```python
from build123d import *

# Parameters (mm, degrees)
F5_DEPTH  = 5
F3_R      = 20
F2_R      = 25
F2_R_2    = 20
F6_DEPTH  = 50
F7_DEPTH  = 10
F0_R      = 5
F0_R_2    = 2.5
F8_DEPTH  = 5
F9_DEPTH  = 25
F10_R     = 17.5
F11_DEPTH = 40
F12_DEPTH = 5
F13_R     = 5
F14_R     = 5


with BuildPart() as f5:
    # F1 (on Top) → F5 (new body)
    with BuildSketch(Plane.XY):
        with BuildLine():
            ThreePointArc((55.0272203653, -51.5364989145), (41.1164714576, 9.8481618987), (0, 57.5033955377))
            ThreePointArc((0, 57.5033955377), (-41.1164714576, 9.8481618987), (-55.0272203653, -51.5364989145))
            ThreePointArc((-55.0272203653, -51.5364989145), (0, -63.7570226936), (55.0272203653, -51.5364989145))
        make_face()
        with BuildLine():
            ThreePointArc((-45, -45), (-32.3889723065, 4.9444861533), (0, 45))
            ThreePointArc((0, 45), (32.3889723065, 4.9444861533), (45, -45))
            ThreePointArc((45, -45), (0, -53.7570226936), (-45, -45))
        make_face(mode=Mode.SUBTRACT)
        with BuildLine():
            ThreePointArc((45, -45), (32.3889723065, 4.9444861533), (0, 45))
            ThreePointArc((0, 45), (-32.3889723065, 4.9444861533), (-45, -45))
            ThreePointArc((-45, -45), (0, -53.7570226936), (45, -45))
        make_face()
    extrude(amount=F5_DEPTH)

    # F3 (on Top) + F2 (on Top) → F6 (join)
    with BuildSketch(Plane.XY):
        with Locations((0, 6.2429773064)):
            Circle(F3_R)
    with BuildSketch(Plane.XY):
        with Locations((0, -23.7570226936)):
            Circle(F2_R)
        with Locations((0, -23.7570226936)):
            Circle(F2_R_2, mode=Mode.SUBTRACT)
        with Locations((0, -23.7570226936)):
            Circle(F2_R_2)
    extrude(amount=F6_DEPTH)

    # F4 (on Top) → F7 (join)
    with BuildSketch(Plane.XY):
        Polygon((52.5, -37.5), (0, -37.5), (-52.5, -37.5), (-52.5, -52.5), (52.5, -52.5), align=None)
        Polygon((-7.5, 10.6258387864), (0, 10.6258387864), (7.5, 10.6258387864), (7.5, 50.6258387864), (-7.5, 50.6258387864), align=None)
    extrude(amount=F7_DEPTH)

    # F0 (on Top) → F8 (cut)
    with BuildSketch(Plane.XY):
        with Locations((-45, -45)):
            Circle(F0_R)
        with Locations((-45, -45)):
            Circle(F0_R_2, mode=Mode.SUBTRACT)
        with Locations((0, 45)):
            Circle(F0_R)
        with Locations((0, 45)):
            Circle(F0_R_2, mode=Mode.SUBTRACT)
        with Locations((45, -45)):
            Circle(F0_R)
        with Locations((45, -45)):
            Circle(F0_R_2, mode=Mode.SUBTRACT)
    extrude(amount=F8_DEPTH, mode=Mode.SUBTRACT)

    # F0 (on Top) → F9 (cut)
    with BuildSketch(Plane.XY):
        with Locations((-45, -45)):
            Circle(F0_R_2)
        with Locations((0, 45)):
            Circle(F0_R_2)
        with Locations((45, -45)):
            Circle(F0_R_2)
    extrude(amount=F9_DEPTH, mode=Mode.SUBTRACT)

    # F10 (on face) + F2 (on Top) → F11 (cut)
    with BuildSketch(Plane.XY):
        with Locations((0, 6.2429773064)):
            Circle(F10_R)
    with BuildSketch(Plane.XY):
        with Locations((0, -23.7570226936)):
            Circle(F2_R_2)
    extrude(amount=F11_DEPTH, mode=Mode.SUBTRACT)

    # F12 (cut): a face of the model
    f12_faces = [f5.faces().sort_by_distance(p)[0] for p in [
        (0, -12.7665147671, 50),
    ]]
    extrude(f12_faces, amount=-F12_DEPTH, mode=Mode.SUBTRACT)

    # F13
    f13_edges = [f5.edges().sort_by_distance(p)[0] for p in [
        (52.5, -52.5, 7.5),
        (52.5, -37.5, 7.5),
        (55.02722, -51.536499, 2.5),
        (-55.02722, -51.536499, 2.5),
        (-52.5, -52.5, 7.5),
        (-52.5, -37.5, 7.5),
        (-7.5, 50.625839, 7.5),
        (0, 57.503396, 2.5),
        (7.5, 50.625839, 7.5),
    ]]
    fillet(f13_edges, radius=F13_R)

    # F14
    f14_edges = [f5.edges().sort_by_distance(p)[0] for p in [
        (19.138968, 12.04814, 5),
        (-24.779157, -20.441394, 5),
        (24.779157, -20.441394, 5),
        (-19.138968, 12.04814, 5),
        (-16.535946, -5.007023, 25),
        (16.535946, -5.007023, 25),
        (0, 26.242977, 45),
        (0, -48.757023, 45),
    ]]
    fillet(f14_edges, radius=F14_R)


solid = f5.part
```
CAD build for the part. Positions are in the model's coordinates, mm. A direction names the side the tool comes from. Round coordinates to 2 decimals unless told otherwise and drop trailing zeros. Write each loop counter-clockwise with the first axis right and the second up, starting at its lowest first coordinate (ties: lowest second). Pieces come first, ordered by that corner, then holes. Notation, with made-up numbers: M 68,-3 L 78,-3 A21 cw 78,15 Z; hole C 49.5,15.25 d1. An arc over 180 degrees is marked long. One line per question, with ' | ' between items.
1. Probe L1, parallel to X at y = -45, z = 8; L2, parallel to Y at x = 0, z = 1; L3, parallel to Y at x = 0, z = 8.95. List the from-to ranges inside material, lowest first. Write a range as from..to.
Working result:
L1: -52.5..-47.5, -42.5..42.5, 47.5..52.5 | L2: -63.76..-43.76, 23.74..40, 50..56.32 | L3: -52.5..-43.76, 23.74..42.5, 47.5..50.63
2. Which spindle directions (+Z, -Z, +X, -X, +Y, -Y) get a long thin tool onto all of the face, cutting with end or side? Do faces 4 (the cylindrical face through (41, -42, 2)), 5 (the cylindrical face through (51, -51.07, 7.54)), 6 (the cylindrical face through (-0.799, -48.744, 24.79)), 7 (the cylindrical face through (-5.996, 49.2, 7.535)), 8 (the cylindrical face through (-51.07, -51, 7.54)). Say none if no direction does.
Working result:
face 4: -Z | face 5: +Z, +X, -Y | face 6: +Z | face 7: +Z, -X, +Y | face 8: +Z, -X, -Y
3. Cut at B-B on x = -32.5. Write the cut outline in (y, z), and give its area (3 significant figures).
Working result:
outline: M -59.63,0 L 24.46,0 L 24.46,5 L -37.5,5 L -37.5,10 L -52.5,10 L -52.5,5 L -59.63,5 Z | area: 495 mm2
4. Mould opens along Y. For faces 1 (the flat face through (-7.5, 35, 7)), 2 (the cylindrical face through (-51, -38.93, 7.54)), 3 (the flat face through (34, -37.5, 7)) say: pulls with the +Y half, pulls with the -Y half, needs draft (parallel to the pull), parting line crosses it, or undercut.
Working result:
face 1: needs draft | face 2: pulls with the +Y half | face 3: undercut
5. Pin check, flat tips, straight feed: pin 1 Ø12 at (x, y) = (2, -19) entering from -Z; pin 2 Ø6 at (x, y) = (-45, -45) entering from -Z; pin 3 Ø2 at (x, z) = (-13.5, 28.5) entering from +Y; pin 4 Ø3 at (x, y) = (-45, -45) entering from -Z. Stop position of each tip, or through.
Working result:
pin 1: z = 40 | pin 2: z = 5 | pin 3: y = 21.86 | pin 4: through
6. Cut at A-A on x = -45. Write the cut outline in (y, z), and give its area (3 significant figures).
Working result:
outline: M -55.72,0 L -50,0 L -50,5 L -47.5,5 L -47.5,10 L -52.5,10 L -52.5,5 L -55.72,5 Z; M -42.5,5 L -40,5 L -40,0 L 1.42,0 L 1.42,5 L -37.5,5 L -37.5,10 L -42.5,10 Z | area: 286 mm2
